Can you work these out from the model? Positions are in its coordinate system, mm. Round coordinates to 2 decimals unless told otherwise and drop trailing zeros. Write each loop counter-clockwise with the first axis right and the second up, starting at its lowest first coordinate (ties: lowest second). Pieces come first, ordered by that corner, then holes. Notation, with made-up numbers: M -11.5,41 L 21.5,41 A22 cw 21.5,48 Z; hole C -34.5,59 d3. An arc over 180 degrees is marked long. Answer as a JSON object with one key per item and string values. Group by question number.
1) Please list where these lines run through material, in increasing order: L1, parallel to Y at x = 0, z = 5; L2, parallel to X at y = 45, z = 9.25; L3, parallel to X at y = 49, z = 4.75. Write a range as [from, to].
2) I'm going to push flat-ended pins straight in: pin 1 Ø6 at (y, z) = (7, 8) entering from +X; pin 2 Ø6 at (y, z) = (-15, 4) entering from -X; pin 3 Ø2 at (y, z) = (47.5, 2) entering from +X. Where does each tip first touch, or does it pass through?
3) Suppose I cut it at B-B, the plane y = 46. Write out the boundary of the cut face in (x, z).
4) Suppose I cut it at A-A, the plane x = 0. Write out the boundary of the cut face in (y, z).
5) Suppose I cut it at C-C, the plane z = 3. Write out the boundary of the cut face in (x, y).
6) Suppose I cut it at D-D, the plane y = -50. Write out the boundary of the cut face in (x, z), and give its area (3 significant figures).
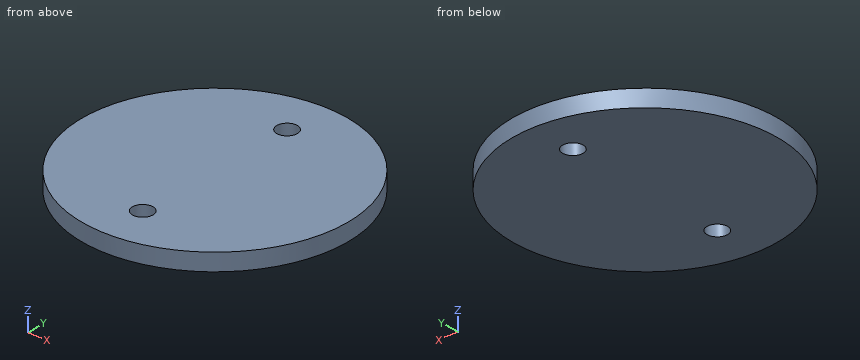
from build123d import *

# Parameters (mm, degrees)
SKETCH_R           = 77
PAD_DEPTH          = 10
SKETCH001_R        = 6
POCKET_DEPTH       = 446.037696
POLARPATTERN_COUNT = 2


with BuildPart() as part:
    # Sketch → Pad (new body)
    with BuildSketch(Plane.XY):
        Circle(SKETCH_R)
    extrude(amount=PAD_DEPTH)

    # Sketch001 (on Face3 of Pad) → Pocket (cut, through all)
    with BuildSketch(Plane.XY.offset(10)):
        with Locations((0, 50)):
            Circle(SKETCH001_R)
    pocket = extrude(amount=-POCKET_DEPTH, mode=Mode.SUBTRACT)

    # PolarPattern: Pocket ×2 about axis
    polarpattern_axis = Axis((0, 0, 10), (0, 0, 1))
    for i in range(1, POLARPATTERN_COUNT):
        add(pocket.rotate(polarpattern_axis, i * 360 / POLARPATTERN_COUNT), mode=Mode.SUBTRACT)


solid = part.part
Results:
{
 "1": {"L1": "[-77, -56], [-44, 44], [56, 77]", "L2": "[-62.48, -3.32], [3.32, 62.48]", "L3": "[-59.4, -5.92], [5.92, 59.4]"},
 "2": {"pin 1": "x = 76.9", "pin 2": "x = -76.06", "pin 3": "x = 61.37"},
 "3": {"outline": "M -61.75,0 L -4.47,0 L -4.47,10 L -61.75,10 Z; M 4.47,0 L 61.75,0 L 61.75,10 L 4.47,10 Z"},
 "4": {"outline": "M -77,0 L -56,0 L -56,10 L -77,10 Z; M -44,0 L 44,0 L 44,10 L -44,10 Z; M 56,0 L 77,0 L 77,10 L 56,10 Z"},
 "5": {"outline": "C 0,0 d154; hole C 0,-50 d12; hole C 0,50 d12"},
 "6": {"outline": "M -58.56,0 L -6,0 L -6,10 L -58.56,10 Z; M 6,0 L 58.56,0 L 58.56,10 L 6,10 Z", "area": "1,050 mm^2"}
}
